```python
from build123d import *

# Parameters (mm, degrees)
BASE_FLANGE1_DEPTH       = 3.2
EDGE_FLANGE17_DEPTH      = 538.435133562
EDGE_FLANGE17_BEND_DEPTH = 537.697496226
EDGE_FLANGE18_DEPTH      = 353.722345428
EDGE_FLANGE18_BEND_DEPTH = 353.043116027


# Sheet-metal steps are written as plain solids
with BuildPart() as part:
    # Sketch1 → Base-Flange1 (new body)
    with BuildSketch(Plane(origin=(0, 0, 0), x_dir=(1, 0, 0), z_dir=(0, 1, 0))):
        Polygon((537.697496226, 353.042345428), (0, 353.042345428), (-0.737637336, 353.042345428), (0, 0), (537.697496226, 0), align=None)
    extrude(amount=-BASE_FLANGE1_DEPTH)

    # Edge-Flange17 section (across the edge) → Edge-Flange17 (add)
    with BuildSketch(Plane(origin=(-0.737637336, -3.2, -354.118945428), x_dir=(0, 0, 1), z_dir=(1, 0, 0))):
        with BuildLine():
            Line((-3.2, 0.7366), (-3.2, 16.15))
            Line((-3.2, 16.15), (0, 16.15))
            Line((0, 16.15), (0, 0.7366))
            ThreePointArc((0, 0.7366), (0.215745145, 0.215745145), (0.7366, 0))
            Line((0.7366, 0), (1.0766, 0))
            Line((1.0766, 0), (1.0766, -3.2))
            Line((1.0766, -3.2), (0.7366, -3.2))
            ThreePointArc((0.7366, -3.2), (-2.046996555, -2.046996555), (-3.2, 0.7366))
        make_face()
    extrude(amount=EDGE_FLANGE17_DEPTH)

    # Edge-Flange17 section 2 (across the edge) → Edge-Flange17 bend (add)
    with BuildSketch(Plane(origin=(537.697496226, -3.2, 1.0766), x_dir=(0, 0, -1), z_dir=(-1, 0, 0))):
        with BuildLine():
            Line((-3.2, 0.7366), (-3.2, 16.15))
            Line((-3.2, 16.15), (0, 16.15))
            Line((0, 16.15), (0, 0.7366))
            ThreePointArc((0, 0.7366), (0.215745145, 0.215745145), (0.7366, 0))
            Line((0.7366, 0), (1.0766, 0))
            Line((1.0766, 0), (1.0766, -3.2))
            Line((1.0766, -3.2), (0.7366, -3.2))
            ThreePointArc((0.7366, -3.2), (-2.046996555, -2.046996555), (-3.2, 0.7366))
        make_face()
    extrude(amount=EDGE_FLANGE17_BEND_DEPTH)

    # Edge-Flange18 section (across the edge) → Edge-Flange18 (add)
    with BuildSketch(Plane(origin=(539.094096226, -3.2, -353.382345428), x_dir=(-1, 0, 0), z_dir=(0, 0, 1))):
        with BuildLine():
            Line((-3.2, 0.7366), (-3.2, 16.15))
            Line((-3.2, 16.15), (0, 16.15))
            Line((0, 16.15), (0, 0.7366))
            ThreePointArc((0, 0.7366), (0.215745145, 0.215745145), (0.7366, 0))
            Line((0.7366, 0), (1.3966, 0))
            Line((1.3966, 0), (1.3966, -3.2))
            Line((1.3966, -3.2), (0.7366, -3.2))
            ThreePointArc((0.7366, -3.2), (-2.046996555, -2.046996555), (-3.2, 0.7366))
        make_face()
    extrude(amount=EDGE_FLANGE18_DEPTH)

    # Edge-Flange18 section 2 (across the edge) → Edge-Flange18 bend (add)
    with BuildSketch(Plane(origin=(-1.396596952, -3.2, 0.002918013), x_dir=(0.999997817266246, -3.4914813388431337e-15, -0.0020893689821821237), z_dir=(-0.0020893689821821237, 0, -0.999997817266246))):
        with BuildLine():
            Line((-3.2, 0.7366), (-3.2, 16.15))
            Line((-3.2, 16.15), (0, 16.15))
            Line((0, 16.15), (0, 0.7366))
            ThreePointArc((0, 0.7366), (0.215745145, 0.215745145), (0.7366, 0))
            Line((0.7366, 0), (1.3966, 0))
            Line((1.3966, 0), (1.3966, -3.2))
            Line((1.3966, -3.2), (0.7366, -3.2))
            ThreePointArc((0.7366, -3.2), (-2.046996555, -2.046996555), (-3.2, 0.7366))
        make_face()
    extrude(amount=EDGE_FLANGE18_BEND_DEPTH)


solid = part.part
```
The listing builds one solid part. Answer for the finished solid, in the listing's coordinates (mm). A direction names the side the tool comes from. Coordinates: 2 decimals unless noted, no trailing zeros. Write each loop counter-clockwise with the first axis right and the second up, starting at its lowest first coordinate (ties: lowest second). Pieces come first, ordered by that corner, then holes. Notation, with made-up numbers: (67, -6.5) -> (125, -6.5) arc R10 ccw to (125, 8.5) -> close; hole circle Ø7 at (46.25, -40). An arc over 180 degrees is marked (long way). Write each question's results on one line, items separated by ' | '. Start each with the question number.
1) Flat-ended cylindrical pins translate along their axes: pin 1 Ø2.5 at (x, y) = (541, -12.5) entering from -Z; pin 2 Ø4.5 at (y, z) = (-6, 2) entering from -X; pin 3 Ø10 at (x, z) = (350, -198) entering from -Y; pin 4 Ø10 at (x, y) = (210, -3) entering from -Z. Find the tip coordinate at first contact, or state that the pin passes through.
2) A cutting plane is placed at B-B (x = 213.5). Determine the outline of the cut face in (y, z).
3) A tool of negligible diameter and unlimited length cuts with its end or side. For faces 4 (the flat face through (265, -12, -354.119)), 5 (the flat face through (265, -12, -357.319)), 6 (the flat face through (539.094, -12, -179)), from which of +Z, -Z, +X, -X, +Y, -Y can it reach the whole face along a straight path? Write none if from no direction.
4) A cutting plane is placed at A-A (y = -15). Determine the outline of the cut face in (x, z).
5) Straight lines are drawn through the part: probe 1 along Z at (x, y) = (96, -6.25); probe 2 along X at (y, z) = (-14.75, -57); probe 3 along X at (y, z) = (-13.5, -320). For each, find the intervals that lie inside material, in ascending order.
6) For a pull along X with two mould halves and no side action, classify faces 1 (the flat face through (542.294, -12, -179)), 2 (the flat face through (265, -3.2, -174)), 3 (the flat face through (273, 0, -174)) as +X half, -X half, draft (parallel to the pull), parting line (faces both ways), or undercut.
Values follow:
1) pin 1: z = -353.38 | pin 2: x = -4.6 | pin 3: y = -3.2 | pin 4: z = -357.32
2) outline: (-19.35, -357.32) -> (-3.94, -357.32) arc R3.94 ccw to (0, -353.38) -> (0, 0.34) arc R3.94 ccw to (-3.94, 4.28) -> (-19.35, 4.28) -> (-19.35, 1.08) -> (-3.94, 1.08) arc R0.74 cw to (-3.2, 0.34) -> (-3.2, -353.38) arc R0.74 cw to (-3.94, -354.12) -> (-19.35, -354.12) -> close
3) face 4: +X, -X, -Y | face 5: -Z, +X, -X, +Y, -Y | face 6: +Z, -Z, -Y
4) outline: (-5.33, -353.03) -> (-2.13, -353.04) -> (-1.4, 0) -> (-4.6, 0.01) -> close; (-0.74, -357.32) -> (537.7, -357.32) -> (537.7, -354.12) -> (-0.74, -354.12) -> close; (0, 1.08) -> (537.7, 1.08) -> (537.7, 4.28) -> (0, 4.28) -> close; (539.09, -353.38) -> (542.29, -353.38) -> (542.29, 0.34) -> (539.09, 0.34) -> close
5) probe 1: -357.32 to -354.12, 1.08 to 4.28 | probe 2: -4.72 to -1.52, 539.09 to 542.29 | probe 3: -5.27 to -2.07, 539.09 to 542.29
6) face 1: +X half | face 2: undercut | face 3: draft
